Work out the finished part from the listing and answer in its coordinate system (mm). A direction names the side the tool comes from. Coordinates: 2 decimals unless noted, no trailing zeros. Order: outer loops, then holes, each group sorted by start corner. A loop starts at its lowest first (then second) coordinate and runs counter-clockwise, first axis right, second up. Notation, with made-up numbers: (34, 14) -> (85, 14) arc R30 cw to (85, 45) -> close; hole circle Ø3 at (-39, -9.5). An arc over 180 degrees is marked (long way). Write item = value, one per line. Start each with the question number.
Q1. The part is cut by section A-A, the plane x = 0. Determine the outline of the cut face in (y, z).
Q2. Which of the six approach directions +Z, -Z, +X, -X, +Y, -Y give full straight-line access (tool end or side, diameter ignored) to faces 4 (the flat face through (0, 83, 25.4)), 5 (the flat face through (0, 25.4, 0)), 6 (the flat face through (0, 83, -25.4))?
Q3. For a pull along X with two mould halves and no side action, classify faces 1 (the cylindrical face through (32.126, 53.35, 20.482)), 2 (the flat face through (0, 25.4, 30)), 3 (the cylindrical face through (3.414, 132.354, 0.356)) as +X half, -X half, draft (parallel to the pull), parting line (faces both ways), or undercut.
Q4. The part is cut by section C-C, the plane z = 0. Determine the outline of the cut face in (x, y).
Q5. The part is cut by section B-B, the plane y = 127. Determine the outline of the cut face in (x, z), plus the area to 3 significant figures.
Q6. Straight lines are drawn through the part: L1, parallel to X at y = 19, z = 0; L2, parallel to Y at x = 0, z = -2; L3, parallel to Z at x = -13, y = 70. For each, find the intervals that lie inside material, in ascending order. Write a range as from..to.
Q7. The part is cut by section D-D, the plane y = 32.5. Determine the outline of the cut face in (x, z), plus the area to 3 significant figures.
Q8. Flat-ended cylindrical pins translate along their axes: pin 1 (10 mm diameter, centred on x = 6, z = -31.5, fed in from +Y); pin 2 (10 mm diameter, centred on x = 0, y = 127, fed in from -Z); pin 3 (5 mm diameter, centred on x = 9.5, y = 30, fed in from +Z); pin 4 (4 mm diameter, centred on y = 93, z = 2.5, fed in from -X). Find the tip coordinate at first contact, or state that the pin passes through.
```python
from build123d import *

# Parameters (mm, degrees)
SKETCH1_R           = 38.1
BOSS_EXTRUDE1_DEPTH = 139.7
SKETCH2_R           = 6.35
CUT_EXTRUDE1_DEPTH  = 25.4
CUT_EXTRUDE2_START  = 25.4
SKETCH3_W           = 76.2
SKETCH3_H           = 114.3
CUT_EXTRUDE2_DEPTH  = 25.4
CUT_EXTRUDE3_START  = -25.4
SKETCH3_2_W         = 76.2
SKETCH3_2_H         = 114.3
CUT_EXTRUDE3_DEPTH  = 25.4
SKETCH4_R           = 6.35
CUT_EXTRUDE4_DEPTH  = 159.113724894


with BuildPart() as part:
    # Sketch1 → Boss-Extrude1 (new body)
    with BuildSketch(Plane(origin=(0, 0, 0), x_dir=(1, 0, 0), z_dir=(0, 1, 0))):
        with Locations(Location((0, 0, 0), (0, 0, 270))):
            Circle(SKETCH1_R)
    extrude(amount=BOSS_EXTRUDE1_DEPTH)

    # Sketch2 → Cut-Extrude1 (cut)
    with BuildSketch(Plane.XZ):
        with Locations(Location((0, 0, 0), (0, 0, 270))):
            Circle(SKETCH2_R)
    extrude(amount=-CUT_EXTRUDE1_DEPTH, mode=Mode.SUBTRACT)

    # Sketch3 → Cut-Extrude2 (cut)
    with BuildSketch(Plane.XY.offset(CUT_EXTRUDE2_START)):
        with Locations((0, 82.55)):
            Rectangle(SKETCH3_W, SKETCH3_H)
    extrude(amount=CUT_EXTRUDE2_DEPTH, mode=Mode.SUBTRACT)

    # Sketch3_2 → Cut-Extrude3 (cut)
    with BuildSketch(Plane.XY.offset(CUT_EXTRUDE3_START)):
        with Locations((0, 82.55)):
            Rectangle(SKETCH3_2_W, SKETCH3_2_H)
    extrude(amount=-CUT_EXTRUDE3_DEPTH, mode=Mode.SUBTRACT)

    # Sketch4 → Cut-Extrude4 (cut, through all)
    with BuildSketch(Plane.XY.offset(25.4)):
        with Locations((0, 127)):
            Circle(SKETCH4_R)
    extrude(amount=-CUT_EXTRUDE4_DEPTH, mode=Mode.SUBTRACT)


solid = part.part
```
Model answer:
q1.outline = (0, -38.1) -> (25.4, -38.1) -> (25.4, -25.4) -> (120.65, -25.4) -> (120.65, 25.4) -> (25.4, 25.4) -> (25.4, 38.1) -> (0, 38.1) -> (0, 6.35) -> (25.4, 6.35) -> (25.4, -6.35) -> (0, -6.35) -> close; (133.35, -25.4) -> (139.7, -25.4) -> (139.7, 25.4) -> (133.35, 25.4) -> close
q2.face_4 = +Z, +X, -X, +Y
q2.face_5 = -Y
q2.face_6 = -Z, +X, -X, +Y
q3.face_1 = parting line
q3.face_2 = draft
q3.face_3 = undercut
q4.outline = (-38.1, 0) -> (-6.35, 0) -> (-6.35, 25.4) -> (6.35, 25.4) -> (6.35, 0) -> (38.1, 0) -> (38.1, 139.7) -> (-38.1, 139.7) -> close; hole circle Ø12.7 at (0, 127)
q5.outline = (-28.4, -25.4) -> (-6.35, -25.4) -> (-6.35, 25.4) -> (-28.4, 25.4) arc R38.1 ccw to start; (6.35, -25.4) -> (28.4, -25.4) arc R38.1 ccw to (28.4, 25.4) -> (6.35, 25.4) -> close
q5.area = 2,920 mm2
q6.L1 = -38.1..-6.35, 6.35..38.1
q6.L2 = 25.4..120.65, 133.35..139.7
q6.L3 = -25.4..25.4
q7.outline = (-28.4, -25.4) -> (28.4, -25.4) arc R38.1 ccw to (28.4, 25.4) -> (-28.4, 25.4) arc R38.1 ccw to start
q7.area = 3,560 mm2
q8.pin_1 = 25.4
q8.pin_2 = through
q8.pin_3 = 25.4
q8.pin_4 = -38.1
